from build123d import *

# Parameters (mm, degrees)
SKETCH_W          = 20
SKETCH_H          = 4
PAD_DEPTH         = 162.5
PAD001_DEPTH      = 20
SKETCH002_R       = 2.5
POCKET_DEPTH      = 0.001
POCKET_DEPTH_BACK = -12.001


with BuildPart() as part:
    # Sketch → Pad (new body, symmetric)
    with BuildSketch(Plane.XZ):
        with Locations((0, 8.9)):
            Rectangle(SKETCH_W, SKETCH_H)
    extrude(amount=PAD_DEPTH, both=True)

    # Sketch001 → Pad001 (join, symmetric)
    with BuildSketch(Plane.YZ):
        Polygon((150.5, 12), (150.5, 0), (174.5, 0), (174.5, 1.5), (162.5, 1.5), (162.5, 12), align=None)
        Polygon((-162.5, 12), (-162.5, 1.5), (-174.5, 1.5), (-174.5, 0), (-150.5, 0), (-150.5, 12), align=None)
    extrude(amount=PAD001_DEPTH, both=True)

    # Sketch002 → Pocket (cut, two sides)
    with BuildSketch(Plane.XY) as pocket_sk:
        with Locations((0, -168.5)):
            Circle(SKETCH002_R)
        with Locations((0, 168.5)):
            Circle(SKETCH002_R)
    extrude(amount=-POCKET_DEPTH, mode=Mode.SUBTRACT)
    extrude(pocket_sk.sketch, amount=-POCKET_DEPTH_BACK, mode=Mode.SUBTRACT)


solid = part.part
Build history of the part. All positions in model axes, mm. A direction names the side the tool comes from. Give positions to 0.01 mm unless a question says otherwise; leave off trailing zeros. Order: outer loops, then holes, each group sorted by start corner. A loop starts at its lowest first (then second) coordinate and runs counter-clockwise, first axis right, second up. Notation, with made-up numbers: M 31,58.5 L 73,58.5 A35 cw 73,92.5 Z; hole C 31.5,11.25 d10. An arc over 180 degrees is marked long. Use one line per item in the form item = value.
Q1. Wall check: probe 1 along Y at (x, z) = (0, 1.05); probe 2 along Y at (x, z) = (11, 6.5); probe 3 along X at (y, z) = (168.5, 0.55). Give the ranges that are in metal, low to high.
Conclusion:
probe_1 = -174.5 to -171, -166 to -150.5, 150.5 to 166, 171 to 174.5
probe_2 = -162.5 to -150.5, 150.5 to 162.5
probe_3 = -20 to -2.5, 2.5 to 20
Q2. Which spindle directions (+Z, -Z, +X, -X, +Y, -Y) get a long thin tool onto all of the face, cutting with end or side? Do faces 5 (the flat face through (-0.3, 171.3, 1.5)), 6 (the flat face through (0, -2, 10.9)), 7 (the flat face through (-20, 157, 6)), 8 (the flat face through (0.3, -165.7, 1.5)), 9 (the flat face through (0, -2, 6.9)). Say none if no direction does.
Conclusion:
face_5 = +Z, +X, -X, +Y
face_6 = +Z, +X, -X
face_7 = +Z, -Z, -X, +Y, -Y
face_8 = +Z, +X, -X, -Y
face_9 = -Z, +X, -X
Q3. Pin check, flat tips, straight feed: P1, Ø16, axis at x = 3.5, y = 28.5, coming from the -Z side; P2, Ø5, axis at x = 0.5, z = 5.5, coming from the -Y side; P3, Ø2, axis at y = 17.5, z = 10, coming from the +X side; P4, Ø4, axis at x = 0, z = 2.5, coming from the -Y side. Stop position of each tip, or through.
Conclusion:
P1 = 6.9
P2 = -162.5
P3 = 10
P4 = -174.5
Q4. Pull direction Y, two halves, no side cores. Call faces 1 (the flat face through (0, 162.5, 7)), 2 (the flat face through (0, -150.5, 6)), 3 (the flat face through (20, -157, 6)), 4 (the flat face through (0, -162.5, 7)): released by +Y, released by -Y, zero draft, split by the parting line, or undercut.
Conclusion:
face_1 = released by +Y
face_2 = undercut
face_3 = zero draft
face_4 = released by -Y
Q5. Slice it at B-B, the plane y = 58. Write the cut outline in (x, z).
Conclusion:
outline = M -10,6.9 L 10,6.9 L 10,10.9 L -10,10.9 Z
Q6. Slice it at A-A, the plane x = -13.5. Write the cut outline in (y, z), and give its area (3 significant figures).
Conclusion:
outline = M -174.5,0 L -150.5,0 L -150.5,12 L -162.5,12 L -162.5,1.5 L -174.5,1.5 Z; M 150.5,0 L 174.5,0 L 174.5,1.5 L 162.5,1.5 L 162.5,12 L 150.5,12 Z
area = 324 mm2
